Source: CAD feature listing. Evaluate the final solid. Frame: model axes, mm. A direction names the side the tool comes from. Round coordinates to 2 decimals unless told otherwise and drop trailing zeros. Loops run counter-clockwise (first coordinate to the right, second up) from the corner with the lowest first, then second, coordinate; pieces in that order, holes last. Notation, with made-up numbers: (63, 22) - (92, 22) arc R22 ccw to (92, 52) - close; hole circle Ø8 at (15, 47). An arc over 180 degrees is marked (long way). One line per question, with ' | ' between items.
from build123d import *

# Parameters (mm, degrees)
SKETCH_1_W              = 15
SKETCH_1_H              = 15
SKETCH_1_W_2            = 12
SKETCH_1_H_2            = 12
EXTRUDE_1_DEPTH         = 600
SKETCH_3_R              = 2.7
CUT_EXTRUDE_2_DEPTH     = 25
SKETCH_4_R              = 2.7
CUT_EXTRUDE_3_DEPTH     = 20
SKETCH_6_R              = 2.75
CUT_EXTRUDE_5_DEPTH     = 30
SKETCH_7_R              = 5
CUT_EXTRUDE_6_DEPTH     = 10
SKETCH_8_R              = 5
CUT_EXTRUDE_7_DEPTH     = 10
SKETCH_9_R              = 5
CUT_EXTRUDE_8_DEPTH     = 10
HOLE_WIZARD_5_4_5_4_1_D = 5.4
CUT_EXTRUDE_9_REACH     = 17
SKETCH_15_R             = 5


with BuildPart() as part:
    # ｽｹｯﾁ1 → ﾎﾞｽ - 押し出し1 (new body)
    with BuildSketch(Plane.XY):
        Rectangle(SKETCH_1_W, SKETCH_1_H)
        Rectangle(SKETCH_1_W_2, SKETCH_1_H_2, mode=Mode.SUBTRACT)
    extrude(amount=EXTRUDE_1_DEPTH)

    # ｽｹｯﾁ3 → ｶｯﾄ - 押し出し2 (cut)
    with BuildSketch(Plane(origin=(0, 7.5, 0), x_dir=(1, 0, 0), z_dir=(0, 1, 0))):
        with Locations((0, -7.5)):
            Circle(SKETCH_3_R)
        with Locations((0, -592.5)):
            Circle(SKETCH_3_R)
        with Locations((0, -366.5)):
            Circle(SKETCH_3_R)
        with Locations((0, -233.5)):
            Circle(SKETCH_3_R)
    extrude(amount=-CUT_EXTRUDE_2_DEPTH, mode=Mode.SUBTRACT)

    # ｽｹｯﾁ4 → ｶｯﾄ - 押し出し3 (cut)
    with BuildSketch(Plane(origin=(7.5, 0, 0), x_dir=(0, 0, -1), z_dir=(1, 0, 0))):
        with Locations((-536, 0)):
            Circle(SKETCH_4_R)
        with Locations((-501, 0)):
            Circle(SKETCH_4_R)
        with Locations((-99, 0)):
            Circle(SKETCH_4_R)
        with Locations((-64, 0)):
            Circle(SKETCH_4_R)
        with Locations((-132, 0)):
            Circle(SKETCH_4_R)
        with Locations((-195, 0)):
            Circle(SKETCH_4_R)
        with Locations((-50, 0)):
            Circle(SKETCH_4_R)
        with Locations((-550, 0)):
            Circle(SKETCH_4_R)
        with Locations((-405, 0)):
            Circle(SKETCH_4_R)
        with Locations((-468, 0)):
            Circle(SKETCH_4_R)
    extrude(amount=-CUT_EXTRUDE_3_DEPTH, mode=Mode.SUBTRACT)

    # ｽｹｯﾁ6 → ｶｯﾄ - 押し出し5 (cut)
    with BuildSketch(Plane(origin=(0, 7.5, 0), x_dir=(1, 0, 0), z_dir=(0, 1, 0))):
        with Locations((0, -435)):
            Circle(SKETCH_6_R)
        with Locations((0, -415)):
            Circle(SKETCH_6_R)
        with Locations((0, -165)):
            Circle(SKETCH_6_R)
        with Locations((0, -185)):
            Circle(SKETCH_6_R)
    extrude(amount=-CUT_EXTRUDE_5_DEPTH, mode=Mode.SUBTRACT)

    # ｽｹｯﾁ7 → ｶｯﾄ - 押し出し6 (cut)
    with BuildSketch(Plane(origin=(0, 7.5, 0), x_dir=(1, 0, 0), z_dir=(0, 1, 0))):
        with Locations((0, -7.5)):
            Circle(SKETCH_7_R)
        with Locations((0, -165)):
            Circle(SKETCH_7_R)
        with Locations((0, -185)):
            Circle(SKETCH_7_R)
        with Locations((0, -233.5)):
            Circle(SKETCH_7_R)
        with Locations((0, -366.5)):
            Circle(SKETCH_7_R)
        with Locations((0, -415)):
            Circle(SKETCH_7_R)
        with Locations((0, -435)):
            Circle(SKETCH_7_R)
        with Locations((0, -592.5)):
            Circle(SKETCH_7_R)
    extrude(amount=-CUT_EXTRUDE_6_DEPTH, mode=Mode.SUBTRACT)

    # ｽｹｯﾁ8 → ｶｯﾄ - 押し出し7 (cut)
    with BuildSketch(Plane(origin=(7.5, 0, 0), x_dir=(0, 0, -1), z_dir=(1, 0, 0))):
        with Locations((-64, 0)):
            Circle(SKETCH_8_R)
        with Locations((-99, 0)):
            Circle(SKETCH_8_R)
        with Locations((-501, 0)):
            Circle(SKETCH_8_R)
        with Locations((-536, 0)):
            Circle(SKETCH_8_R)
    extrude(amount=-CUT_EXTRUDE_7_DEPTH, mode=Mode.SUBTRACT)

    # ｽｹｯﾁ9 → ｶｯﾄ - 押し出し8 (cut)
    with BuildSketch(Plane.ZY.offset(7.5)):
        with Locations((132, 0)):
            Circle(SKETCH_9_R)
        with Locations((50, 0)):
            Circle(SKETCH_9_R)
        with Locations((195, 0)):
            Circle(SKETCH_9_R)
        with Locations((405, 0)):
            Circle(SKETCH_9_R)
        with Locations((550, 0)):
            Circle(SKETCH_9_R)
        with Locations((468, 0)):
            Circle(SKETCH_9_R)
    extrude(amount=-CUT_EXTRUDE_8_DEPTH, mode=Mode.SUBTRACT)

    # Ø5.4 (5.4) 直径の穴1 (through all)
    with Locations(Plane(origin=(0, -7.5, 0), x_dir=(-1, 0, 0), z_dir=(0, -1, 0))):
        with Locations((0, -252.5), (0, -347.5)):
            Hole(HOLE_WIZARD_5_4_5_4_1_D / 2)

    # ｽｹｯﾁ15 → ｶｯﾄ - 押し出し9 (cut, up to next)
    with BuildSketch(Plane(origin=(0, 7.5, 0), x_dir=(1, 0, 0), z_dir=(0, 1, 0)), mode=Mode.PRIVATE) as cut_extrude_9_sk1:
        with Locations((0, -252.5)):
            Circle(SKETCH_15_R)
    cut_extrude_9_tool1 = extrude(cut_extrude_9_sk1.sketch, amount=-CUT_EXTRUDE_9_REACH, mode=Mode.PRIVATE) & part.part
    add(cut_extrude_9_tool1.solids().sort_by_distance((0, 7.5, 252.5))[0], mode=Mode.SUBTRACT)
    # ｽｹｯﾁ15 → ｶｯﾄ - 押し出し9 (cut, up to next)
    with BuildSketch(Plane(origin=(0, 7.5, 0), x_dir=(1, 0, 0), z_dir=(0, 1, 0)), mode=Mode.PRIVATE) as cut_extrude_9_sk2:
        with Locations((0, -347.5)):
            Circle(SKETCH_15_R)
    cut_extrude_9_tool2 = extrude(cut_extrude_9_sk2.sketch, amount=-CUT_EXTRUDE_9_REACH, mode=Mode.PRIVATE) & part.part
    add(cut_extrude_9_tool2.solids().sort_by_distance((0, 7.5, 347.5))[0], mode=Mode.SUBTRACT)


solid = part.part
1. Mould query, pull axis Z, two halves, no side actions, for faces 4 (the flat face through (-7, 0, 600)), 5 (the cylindrical face through (-0.651, 6.76, 587.543)), 6 (the flat face through (0, 6, 296)). Classes: released by +Z, released by -Z, zero draft, split by the parting line, or undercut.
Worked out:
face 4: released by +Z | face 5: undercut | face 6: zero draft
2. Access query for faces 1 (the cylindrical face through (-7, -3, 191)), 2 (the cylindrical face through (7, 0, 69)), 3 (the cylindrical face through (-0.651, 6.76, 228.543)). Directions: +Z, -Z, +X, -X, +Y, -Y. A direction counts if a zero-diameter tool reaches every point of the face in a straight line with its end or side. Return the directions, or none.
Worked out:
face 1: -X | face 2: +X | face 3: +Y
3. Material intervals for probe 1 along Y at (x, z) = (4.25, 522); probe 2 along Y at (x, z) = (7, 536), sorted ascending.
Worked out:
probe 1: y = -7.5 to -6, 6 to 7.5 | probe 2: y = -7.5 to -5, 5 to 7.5
4. Section query A-A, the plane z = 391. Return loops of the section in (x, y).
Worked out:
outline: (-7.5, -7.5) - (7.5, -7.5) - (7.5, 7.5) - (-7.5, 7.5) - close; hole (-6, -6) - (6, -6) - (6, 6) - (-6, 6) - close
5. Contact query for flat-ended pins moving along their axis: P1, Ø5, axis at x = 0, z = 415, coming from the -Y side; P2, Ø8, axis at x = 0, z = 185, coming from the +Y side; P3, Ø6, axis at y = 0, z = 536, coming from the +X side. Output: stop coordinate, or through.
Worked out:
P1: passes through | P2: stops at y = -6 | P3: stops at x = -6
